Part model, mm, in its own coordinate system. A direction names the side the tool comes from. Coordinates: 2 decimals unless noted, no trailing zeros. Order: outer loops, then holes, each group sorted by start corner. A loop starts at its lowest first (then second) coordinate and runs counter-clockwise, first axis right, second up. Notation, with made-up numbers: (41.5, 20) - (91.5, 20) arc R33 ccw to (91.5, 58) - close; hole circle Ø8 at (-12.5, 16). An arc over 180 degrees is marked (long way). Use a Markdown table: item, result. Add a question column.
1) Tool access for faces 1 (the face through (46.266, -28.465, 63.785)), 2 (the face through (-46.4, -27.8, 66)), 3 (the face through (42.5, -28, 31)), 4 (the face through (50.5, -27, 31)), 5 (the face through (48.115, -19.231, 1.895)): list every direction of +Z, -Z, +X, -X, +Y, -Y with a clear straight run to the whole face (end or side of a thin tool).
2) Saw through at C-C on y = 12.5. List the corners of the cut face in (x, z).
3) Two-plate mould, pull along Y, no slides. Class faces 6 (the face through (-52, -23, 39)), 7 (the face through (-45.669, -28.465, 3.403)), 8 (the face through (46, -26, 64)), 9 (the face through (-50, 0, 40)): +Y half, -Y half, draft (parallel to the pull), parting line (faces both ways), or undercut.
4) Saw through at D-D on x = 46.5. Count the separate pieces of the cut face and the enclosed holes in it, then the cut area to 3 significant figures.
5) Wall check: L1, parallel to Y at x = -39, z = 35; L2, parallel to X at y = -11, z = 28; L3, parallel to Z at x = 46.5, y = -23.3. Give the ranges that are in metal, low to high. Write a range as [from, to].
6) Saw through at A-A on x = 30.5. List the corners of the cut face in (y, z).
7) Saw through at B-B on z = 45.5. List the corners of the cut face in (x, y), then the cut area to 3 significant figures.
8) Drop flat-ended pins along their axis: P1, Ø3, axis at x = -46.5, z = 62, coming from the -Y side; P2, Ø4, axis at x = 46.5, z = 62, coming from the -Y side; P3, Ø6, axis at x = 14.5, z = 70.5, coming from the -Y side; P4, Ø1.7, axis at y = -27, z = 43.5, coming from the +X side. Give the stop position or say it passes through.
```python
from build123d import *

# Parameters (mm, degrees)
F0_W     = 108
F0_H     = 52
F0_W_2   = 100
F0_H_2   = 44
F1_DEPTH = 80
F2_DEPTH = 2
F3_R     = 3.5
F3_R_2   = 1.8
F4_DEPTH = 5
F5_DEPTH = 25
F6_SIZE  = 5
F7_SIZE  = 1
F8_W     = 84
F8_H     = 37
F9_DEPTH = 25


with BuildPart() as f1:
    # F0 (on Top) → F1 (new body)
    with BuildSketch(Plane.XY):
        Rectangle(F0_W, F0_H)
        Rectangle(F0_W_2, F0_H_2, mode=Mode.SUBTRACT)
    extrude(amount=F1_DEPTH)

    # F0 (on Top) → F2 (join)
    with BuildSketch(Plane.XY):
        Rectangle(F0_W_2, F0_H_2)
    extrude(amount=F2_DEPTH)

    # F3 (on face) → F4 (join)
    with BuildSketch(Plane.XZ.offset(26)):
        with BuildLine():
            Line((-42.5, 0), (-42.5, 62))
            ThreePointArc((-42.5, 62), (-46.5, 66), (-50.5, 62))
            Line((-50.5, 62), (-50.5, 0))
            Line((-50.5, 0), (-42.5, 0))
        make_face()
        with Locations((-46.5, 5)):
            Circle(F3_R, mode=Mode.SUBTRACT)
        with Locations((-46.5, 62)):
            Circle(F3_R, mode=Mode.SUBTRACT)
        with BuildLine():
            Line((42.5, 62), (42.5, 0))
            Line((42.5, 0), (50.5, 0))
            Line((50.5, 0), (50.5, 62))
            ThreePointArc((50.5, 62), (46.5, 66), (42.5, 62))
        make_face()
        with Locations((46.5, 5)):
            Circle(F3_R, mode=Mode.SUBTRACT)
        with Locations((46.5, 62)):
            Circle(F3_R, mode=Mode.SUBTRACT)
        with Locations((46.5, 62)):
            Circle(F3_R)
        with Locations((46.5, 62)):
            Circle(F3_R_2, mode=Mode.SUBTRACT)
        with Locations((-46.5, 62)):
            Circle(F3_R)
        with Locations((-46.5, 62)):
            Circle(F3_R_2, mode=Mode.SUBTRACT)
        with Locations((-46.5, 5)):
            Circle(F3_R)
        with Locations((-46.5, 5)):
            Circle(F3_R_2, mode=Mode.SUBTRACT)
        with Locations((46.5, 5)):
            Circle(F3_R)
        with Locations((46.5, 5)):
            Circle(F3_R_2, mode=Mode.SUBTRACT)
    extrude(amount=F4_DEPTH)

    # F3 (on face) → F5 (cut)
    with BuildSketch(Plane.XZ.offset(26)):
        with Locations((-46.5, 5)):
            Circle(F3_R)
        with Locations((-46.5, 5)):
            Circle(F3_R_2, mode=Mode.SUBTRACT)
        with Locations((46.5, 5)):
            Circle(F3_R)
        with Locations((46.5, 5)):
            Circle(F3_R_2, mode=Mode.SUBTRACT)
        with Locations((46.5, 62)):
            Circle(F3_R)
        with Locations((46.5, 62)):
            Circle(F3_R_2, mode=Mode.SUBTRACT)
        with Locations((46.5, 62)):
            Circle(F3_R_2)
        with Locations((46.5, 5)):
            Circle(F3_R_2)
        with Locations((-46.5, 5)):
            Circle(F3_R_2)
        with Locations((-46.5, 62)):
            Circle(F3_R)
        with Locations((-46.5, 62)):
            Circle(F3_R_2, mode=Mode.SUBTRACT)
        with Locations((-46.5, 62)):
            Circle(F3_R_2)
    extrude(amount=-F5_DEPTH, mode=Mode.SUBTRACT)

    # F6
    f6_edges = [f1.edges().sort_by_distance(p)[0] for p in [
        (54, 26, 40),
        (54, -26, 40),
        (-54, -26, 40),
        (-54, 26, 40),
    ]]
    chamfer(f6_edges, length=F6_SIZE)

    # F7
    f7_edges = [f1.edges().sort_by_distance(p)[0] for p in [
        (0, 22, 80),
        (-50, 0, 80),
        (0, -22, 80),
        (50, 0, 80),
        (-42.5, -31, 31),
        (-50.5, -31, 31),
        (42.5, -31, 31),
    ]]
    chamfer(f7_edges, length=F7_SIZE)

    # F8 (on face) → F9 (cut)
    with BuildSketch(Plane.XY.offset(2)):
        Rectangle(F8_W, F8_H)
    extrude(amount=-F9_DEPTH, mode=Mode.SUBTRACT)


solid = f1.part
```
Results are:
| question | item | result |
|---|---|---|
| 1 | face 1 | -Y |
| 1 | face 2 | +Z, -Y |
| 1 | face 3 | +Z, -Z, -Y |
| 1 | face 4 | +Z, -Z, +X, -Y |
| 1 | face 5 | none |
| 2 | outline | (-54, 0) - (-42, 0) - (-42, 2) - (-50, 2) - (-50, 79) - (-51, 80) - (-54, 80) - close; (42, 0) - (54, 0) - (54, 80) - (51, 80) - (50, 79) - (50, 2) - (42, 2) - close |
| 3 | face 6 | -Y half |
| 3 | face 7 | draft |
| 3 | face 8 | undercut |
| 3 | face 9 | undercut |
| 4 | separate pieces | 3 |
| 4 | enclosed holes | 0 |
| 4 | area | 954 mm2 |
| 5 | L1 | [-26, -22], [22, 26] |
| 5 | L2 | [-54, -50], [50, 54] |
| 5 | L3 | [0, 1.5], [8.5, 58.5], [65.5, 80] |
| 6 | outline | (-26, 0) - (-18.5, 0) - (-18.5, 2) - (-22, 2) - (-22, 79) - (-23, 80) - (-26, 80) - close; (18.5, 0) - (26, 0) - (26, 80) - (23, 80) - (22, 79) - (22, 2) - (18.5, 2) - close |
| 7 | outline | (-54, -21) - (-50.5, -24.5) - (-50.5, -30) - (-49.5, -31) - (-43.5, -31) - (-42.5, -30) - (-42.5, -26) - (42.5, -26) - (42.5, -30) - (43.5, -31) - (49.5, -31) - (50.5, -30) - (50.5, -24.5) - (54, -21) - (54, 21) - (49, 26) - (-49, 26) - (-54, 21) - close; hole (-50, -22) - (50, -22) - (50, 22) - (-50, 22) - close |
| 7 | area | 1,250 mm2 |
| 8 | P1 | y = 22 |
| 8 | P2 | y = -31 |
| 8 | P3 | y = -26 |
| 8 | P4 | x = 50.5 |
